Design review of the part shown in the three views and the two pictorial views. Dimensions are in mm from the part's minimum x, y and z. Give positions to 0.01 mm unless a question says otherwise; leave off trailing zeros. Write each loop counter-clockwise with the first axis right and the second up, starting at its lowest first coordinate (ties: lowest second). Pieces come first, ordered by that corner, then holes.
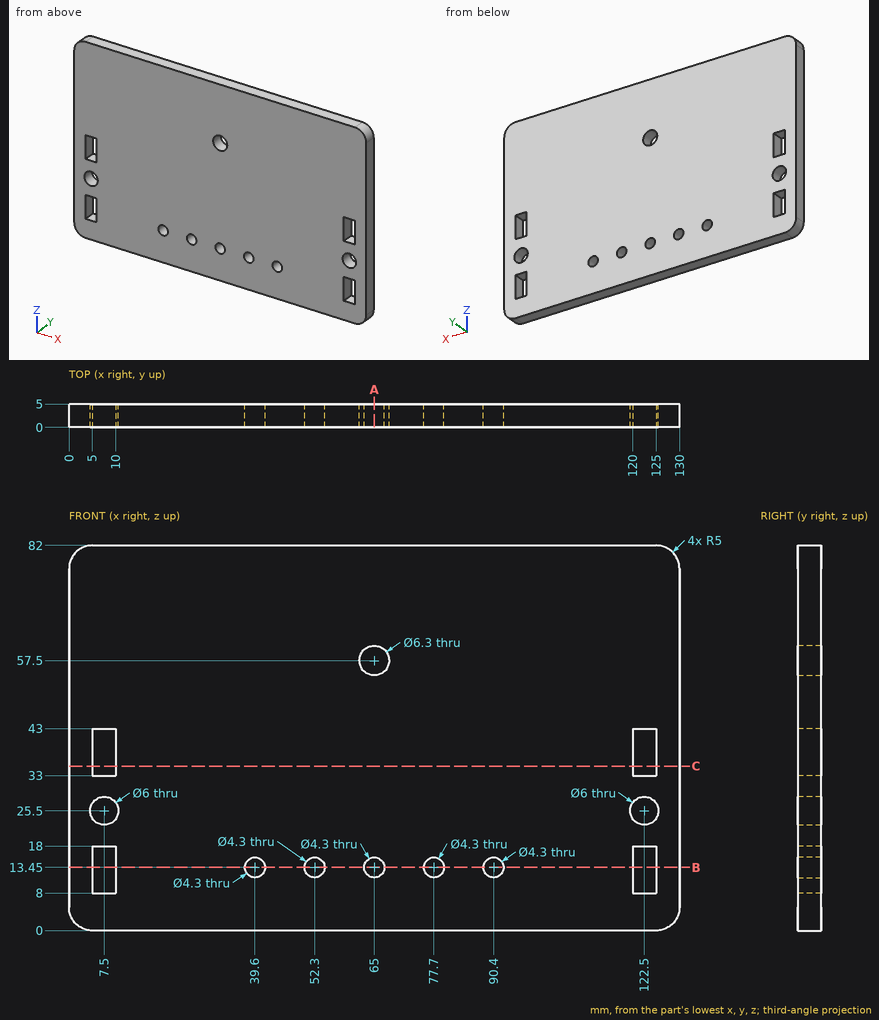
(1) Consider section A-A, the plane x = 65. Give the boundary of the cut face in (y, z).
Resolved:
outline: (0, 0) - (5, 0) - (5, 11.3) - (0, 11.3) - close; (0, 15.6) - (5, 15.6) - (5, 54.35) - (0, 54.35) - close; (0, 60.65) - (5, 60.65) - (5, 82) - (0, 82) - close
(2) Consider section B-B, the plane z = 13.45. Give the number of separate pieces and of enclosed holes in the cut face, then the cut area to 4 significant figures.
Resolved:
separate pieces: 8
enclosed holes: 0
area: 492.5 mm2
(3) To check wall thickness, follow L1, parallel to X at y = 0.8, z = 8.5; L2, parallel to Z at x = 77.5, y = 4.25; L3, parallel to X at y = 1.65, z = 55. State the ranges of each line that lie inside material, in increasing order.
Resolved:
L1: x = 0 to 5, 10 to 120, 125 to 130
L2: z = 0 to 11.31, 15.59 to 82
L3: x = 0 to 63.08, 66.92 to 130
(4) Consider section C-C, the plane z = 35. Give the boundary of the cut face in (x, y), then the cut area to 3 significant figures.
Resolved:
outline: (0, 0) - (5, 0) - (5, 5) - (0, 5) - close; (10, 0) - (120, 0) - (120, 5) - (10, 5) - close; (125, 0) - (130, 0) - (130, 5) - (125, 5) - close
area: 600 mm2
